Build history of the part. All positions in model axes, mm. A direction names the side the tool comes from. Round coordinates to 2 decimals unless told otherwise and drop trailing zeros. Write each loop counter-clockwise with the first axis right and the second up, starting at its lowest first coordinate (ties: lowest second). Pieces come first, ordered by that corner, then holes. Notation, with made-up numbers: M -4,1 L 16,1 A23 ccw 16,20 Z; hole C -6.75,59.5 d6. An arc over 180 degrees is marked long. One line per item, written item: value. Start each with the question number.
```python
from build123d import *

# Parameters (mm, degrees)
SZKIC1_W                    = 21
SZKIC1_H                    = 6
SZKIC1_H_2                  = 20
SZKIC1_R                    = 2.7
DODANIE_WYCI_GNI_CIE1_DEPTH = 6
SZKIC2_W                    = 21
SZKIC2_H                    = 6
DODANIE_WYCI_GNI_CIE2_DEPTH = 20
SZKIC3_R                    = 2.7
WYTNIJ_WYCI_GNI_CIE1_DEPTH  = 9
SZKIC4_W                    = 21
SZKIC4_H                    = 6
DODANIE_WYCI_GNI_CIE3_DEPTH = 14
WYTNIJ_WYCI_GNI_CIE2_DEPTH  = 40.05
SZKIC6_R                    = 4.5
SZKIC6_R_2                  = 2.7
DODANIE_WYCI_GNI_CIE5_DEPTH = 3.7
ZAOKR_GLENIE2_R             = 6
SZKIC7_W                    = 5
SZKIC7_H                    = 18.65
DODANIE_WYCI_GNI_CIE6_DEPTH = 14
ZAOKR_GLENIE3_R             = 6


with BuildPart() as part:
    # Szkic1 → Dodanie-wyciągnięcie1 (new body)
    with BuildSketch(Plane.XY):
        with Locations((10.5, 23)):
            Rectangle(SZKIC1_W, SZKIC1_H)
        with Locations((10.5, 10)):
            Rectangle(SZKIC1_W, SZKIC1_H_2)
        with Locations((8, 10)):
            Circle(SZKIC1_R, mode=Mode.SUBTRACT)
    extrude(amount=DODANIE_WYCI_GNI_CIE1_DEPTH)

    # Szkic2 → Dodanie-wyciągnięcie2 (add)
    with BuildSketch(Plane(origin=(0, 0, 0), x_dir=(-1, 0, 0), z_dir=(0, 0, -1))):
        with Locations((-10.5, 23)):
            Rectangle(SZKIC2_W, SZKIC2_H)
    extrude(amount=DODANIE_WYCI_GNI_CIE2_DEPTH)

    # Szkic3 → Wytnij-wyciągnięcie1 (cut)
    with BuildSketch(Plane(origin=(0, 26, 0), x_dir=(1, 0, 0), z_dir=(0, 1, 0))):
        with Locations((10.5, 10)):
            Circle(SZKIC3_R)
    extrude(amount=-WYTNIJ_WYCI_GNI_CIE1_DEPTH, mode=Mode.SUBTRACT)

    # Szkic4 → Dodanie-wyciągnięcie3 (add)
    with BuildSketch(Plane.XY.offset(6)):
        with Locations((10.5, 21.65)):
            Rectangle(SZKIC4_W, SZKIC4_H)
    extrude(amount=DODANIE_WYCI_GNI_CIE3_DEPTH)

    # Szkic5 → Wytnij-wyciągnięcie2 (cut)
    with BuildSketch(Plane(origin=(0, 24.65, 0), x_dir=(1, 0, 0), z_dir=(0, 1, 0))):
        with BuildLine():
            Line((2.05, -16), (2.05, -10))
            ThreePointArc((2.05, -10), (3.3, -8.75), (4.55, -10))
            Line((4.55, -10), (4.55, -16))
            ThreePointArc((4.55, -16), (3.3, -17.25), (2.05, -16))
        make_face()
        with BuildLine():
            Line((13.65, -16), (13.65, -10))
            ThreePointArc((13.65, -10), (12.4, -8.75), (11.15, -10))
            Line((11.15, -10), (11.15, -16))
            ThreePointArc((11.15, -16), (12.4, -17.25), (13.65, -16))
        make_face()
    extrude(amount=-WYTNIJ_WYCI_GNI_CIE2_DEPTH, mode=Mode.SUBTRACT)

    # Szkic6 → Dodanie-wyciągnięcie5 (add)
    with BuildSketch(Plane(origin=(0, 26, 0), x_dir=(1, 0, 0), z_dir=(0, 1, 0))):
        with Locations((10.5, 10)):
            Circle(SZKIC6_R)
        with Locations((10.5, 10)):
            Circle(SZKIC6_R_2, mode=Mode.SUBTRACT)
    extrude(amount=DODANIE_WYCI_GNI_CIE5_DEPTH)

    # Zaokrąglenie2
    zaokr_glenie2_edges = [part.edges().sort_by_distance(p)[0] for p in [
        (0, 23, -20),
    ]]
    fillet(zaokr_glenie2_edges, radius=ZAOKR_GLENIE2_R)

    # Szkic7 → Dodanie-wyciągnięcie6 (add)
    with BuildSketch(Plane.XY.offset(6)):
        with Locations((18.5, 9.325)):
            Rectangle(SZKIC7_W, SZKIC7_H)
    extrude(amount=DODANIE_WYCI_GNI_CIE6_DEPTH)

    # Zaokrąglenie3
    zaokr_glenie3_edges = [part.edges().sort_by_distance(p)[0] for p in [
        (18.5, 0, 20),
    ]]
    fillet(zaokr_glenie3_edges, radius=ZAOKR_GLENIE3_R)


solid = part.part
```
Item 1: Two-plate mould, pull along Y, no slides. Class faces 1 (the flat face through (8, 18.65, 13)), 2 (the cylindrical face through (12.43, 21.69, 8.75)), 3 (the cylindrical face through (9.452, 12.277, 2.958)): pulls with the +Y half, pulls with the -Y half, needs draft (parallel to the pull), parting line crosses it, or undercut.
Item 2: Cut at B-B, the plane y = 10. Write the cut outline in (x, z).
Item 3: Cut at D-D, the plane z = 0.5. Write the cut outline in (x, y), plus the area to 3 significant figures.
Item 4: Cut at A-A, the plane z = -10. Write the cut outline in (x, y), plus the area to 3 significant figures.
Item 5: Drop flat-ended pins along their axis: pin 1 (7 mm diameter, centred on x = 8, y = 10, fed in from +Z); pin 2 (1.8 mm diameter, centred on y = 20.5, z = 12, fed in from -X); pin 3 (3 mm diameter, centred on x = 10.5, z = -10, fed in from -Y); pin 4 (4 mm diameter, centred on x = 12, z = 15, fed in from -Y). Give the stop position or say it passes through.
Item 6: Which spindle directions (+Z, -Z, +X, -X, +Y, -Y) get a long thin tool onto all of the face, cutting with end or side? Do faces 4 (the flat face through (13, 20, 20)), 5 (the flat face through (10, 7, 6)), 6 (the cylindrical face through (3.33, 21.69, 17.25)), 7 (the flat face through (10, 25, 6)). Say none if no direction does.
Item 7: Drill centre lines: line 1 (X direction, y = 23.1, z = -10); line 2 (Z direction, x = 9.25, y = 3.25); line 3 (Z direction, x = 16.25, y = 7.25). Where is each one in solid material? Low to high.
Item 8: Cut at C-C, the plane x = 3.5. Write the cut outline in (y, z), plus the area to 3 significant figures.
Computed values:
1. face 1: pulls with the -Y half
1. face 2: needs draft
1. face 3: undercut
2. outline: M 0,0 L 5.3,0 L 5.3,6 L 0,6 Z; M 10.7,0 L 21,0 L 21,20 L 16,20 L 16,6 L 10.7,6 Z
3. outline: M 0,0 L 21,0 L 21,26 L 0,26 Z; hole C 8,10 d5.4
3. area: 523 mm2
4. outline: M 0,20 L 7.8,20 L 7.8,29.7 L 6,29.7 L 6,26 L 0,26 Z; M 13.2,20 L 21,20 L 21,26 L 15,26 L 15,29.7 L 13.2,29.7 Z
4. area: 107 mm2
5. pin 1: stops at z = 6
5. pin 2: stops at x = 0
5. pin 3: passes through
5. pin 4: stops at y = 18.65
6. face 4: +Z, +X, -X, +Y, -Y
6. face 5: +Z, -X, -Y
6. face 6: +Y, -Y
6. face 7: +Z, +X, -X, +Y
7. line 1: x = 0 to 7.8, 13.2 to 21
7. line 2: z = 0 to 6
7. line 3: z = 0 to 20
8. outline: M 0,0 L 20,0 L 20,-19.45 L 26,-19.45 L 26,6 L 24.65,6 L 24.65,8.77 L 18.65,8.77 L 18.65,6 L 0,6 Z; M 18.65,17.23 L 24.65,17.23 L 24.65,20 L 18.65,20 Z
8. area: 306 mm2
